```python
from build123d import *

# Parameters (mm, degrees)
SKETCH1_R                    = 4.7625
EXTRUDE1_DEPTH               = 17.78
EXTRUDE2_DEPTH               = 20.01292225
EXTRUDE2_DEPTH_BACK          = 20.01292225
F_1_8_0_125_DIAMETER_HOLE4_D = 3.175


with BuildPart() as part:
    # Sketch1 → Extrude1 (new body)
    with BuildSketch(Plane.XY):
        Circle(SKETCH1_R)
    extrude(amount=EXTRUDE1_DEPTH)

    # Sketch2 → Extrude2 (cut, two sides: drawn at the far end of the back side and taken through both)
    with BuildSketch(Plane(origin=(0, 0, 0), x_dir=(1, 0, 0), z_dir=(0, 1, 0)).offset(-EXTRUDE2_DEPTH_BACK)):
        Polygon((0, 0), (4.7625, -4.7625), (4.7625, 1.90519665), (-4.7625, 1.90519665), (-4.7625, -4.7625), align=None)
    extrude(amount=EXTRUDE2_DEPTH + EXTRUDE2_DEPTH_BACK, mode=Mode.SUBTRACT)

    # 1/8 (0.125) Diameter Hole4 (through all)
    with Locations(Plane(origin=(-4.7625, 0, 17.78), x_dir=(0, 0, 1), z_dir=(-1, 0, 0))):
        with Locations((-7.9502, 0)):
            Hole(F_1_8_0_125_DIAMETER_HOLE4_D / 2)


solid = part.part
```
Design review of the part built by this model. Coordinates are the model's own, in mm. Coordinates: 2 decimals unless noted, no trailing zeros. Order: outer loops, then holes, each group sorted by start corner. A loop starts at its lowest first (then second) coordinate and runs counter-clockwise, first axis right, second up.
1) Take a section at A-A, the plane y = 0. Give the boundary of the cut face in (x, z).
2) Clearance check with flat-ended pins moving along their axes: pin 1 (1.5 mm diameter, centred on y = 2.5, z = 15, fed in from +X); pin 2 (3.5 mm diameter, centred on y = 0, z = 9.83, fed in from -X); pin 3 (3 mm diameter, centred on x = -2, y = 1, fed in from -Z); pin 4 (1.5 mm diameter, centred on y = -1.5, z = 9, fed in from +X). State where each tip first meets the part, or that it passes through.
3) Mouldability with a two-part tool opening along Y and no side actions: class faces 1 (the cylindrical face through (2.56, 4.016, 10.741)), 2 (the flat face through (2, 0, 2)), 3 (the cylindrical face through (0.067, -0.608, 8.363)) as +Y half, -Y half, draft (parallel to the pull), parting line (faces both ways), or undercut.
4) Take a section at D-D, the plane y = -2. Give the boundary of the cut face in (x, z).
5) Wall thickness on line 1 along Z through (x, y) = (-1.25, 0.25); line 2 along Z through (x, y) = (2.25, -0.75); line 3 along X through (y, z) = (4, 7.75): over which ranges is each line inside the solid? List them lowest first.
6) Take a section at C-C, the plane z = 8.5. Give the boundary of the cut face in (x, y) (1 decimal), and give its area (3 significant figures).
Returned:
1. outline: (-4.76, 4.76) - (0, 0) - (4.76, 4.76) - (4.76, 8.24) - (-4.76, 8.24) - close; (-4.76, 11.42) - (4.76, 11.42) - (4.76, 17.78) - (-4.76, 17.78) - close
2. pin 1: stops at x = 4.43
2. pin 2: stops at x = -4.76
2. pin 3: stops at z = 0.5
2. pin 4: stops at x = 4.67
3. face 1: parting line
3. face 2: draft
3. face 3: undercut
4. outline: (-4.32, 4.32) - (0, 0) - (4.32, 4.32) - (4.32, 17.78) - (-4.32, 17.78) - close
5. line 1: z = 1.25 to 8.26, 11.4 to 17.78
5. line 2: z = 2.25 to 8.43, 11.23 to 17.78
5. line 3: x = -2.58 to 2.58
6. outline: (-4.7, -0.9) arc R4.8 ccw to (4.7, -0.9) - close; (-4.7, 0.9) - (4.7, 0.9) arc R4.8 ccw to start
6. area: 54.8 mm2
